Read the model definition and answer for the solid it produces. Units are mm, in the model's axes. Coordinates: 2 decimals unless noted, no trailing zeros. Write each loop counter-clockwise with the first axis right and the second up, starting at its lowest first coordinate (ties: lowest second). Pieces come first, ordered by that corner, then holes.
1) The part is cut by section B-B (x = 0). Determine the outline of the cut face in (y, z), then the cut area to 3 significant figures.
2) The part is cut by section A-A (y = -1.7). Determine the outline of the cut face in (x, z).
3) The part is cut by section D-D (x = 16). Determine the outline of the cut face in (y, z), then the cut area to 3 significant figures.
4) Each of these flat-tipped pins is pushed along its axis until it touches: pin 1 Ø1.1 at (y, z) = (-1.5, 15) entering from -X; pin 2 Ø6 at (x, z) = (-13.5, -16) entering from -Y; pin 3 Ø0.5 at (x, y) = (-0.5, -1) entering from +Z. Where does it stop, or does it pass through?
5) The part is cut by section C-C (z = 0). Determine the outline of the cut face in (x, y).
6) Find the intervals of material crossed by line 1 (Z direction, x = 1, y = -1.75); line 2 (Y direction, x = -15, z = 2); line 3 (X direction, y = 0.35, z = 18.5), in increasing order.
from build123d import *

# Parameters (mm, degrees)
FRONT_W       = 20.95
FRONT_H       = 1
SKETCH1_W     = 4
SKETCH1_H     = 1
HOLDERS_DEPTH = 1.8


with BuildPart() as part:
    # Front → Base (revolve)
    with BuildSketch(Plane.XY, mode=Mode.PRIVATE) as base_sk:
        with Locations((-10.475, 0)):
            Rectangle(FRONT_W, FRONT_H)
    revolve(base_sk.sketch.rotate(Axis((0, 0, 0), (0, 1, 0)), 270), axis=Axis((0, 0, 0), (0, 1, 0)))

    # Sketch1 → Holders (add)
    with BuildSketch(Plane.XZ.offset(0.5)):
        with Locations((0, 15)):
            Rectangle(SKETCH1_W, SKETCH1_H)
        with Locations((0, -15)):
            Rectangle(SKETCH1_W, SKETCH1_H)
    extrude(amount=HOLDERS_DEPTH)


solid = part.part
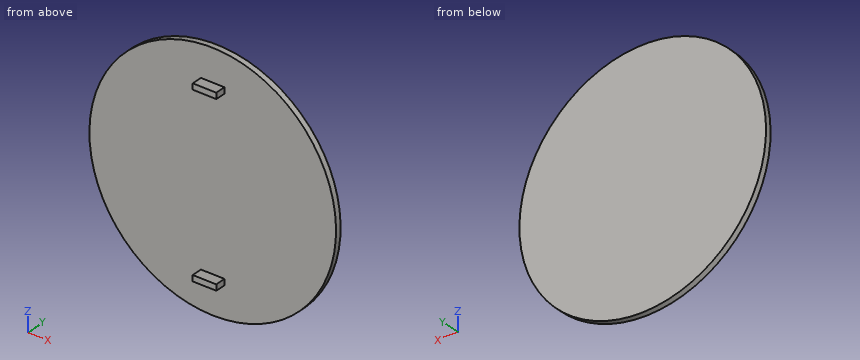
Reported:
1. outline: (-2.3, -15.5) - (-0.5, -15.5) - (-0.5, -20.95) - (0.5, -20.95) - (0.5, 20.95) - (-0.5, 20.95) - (-0.5, 15.5) - (-2.3, 15.5) - (-2.3, 14.5) - (-0.5, 14.5) - (-0.5, -14.5) - (-2.3, -14.5) - close
1. area: 45.5 mm2
2. outline: (-2, -15.5) - (2, -15.5) - (2, -14.5) - (-2, -14.5) - close; (-2, 14.5) - (2, 14.5) - (2, 15.5) - (-2, 15.5) - close
3. outline: (-0.5, -13.52) - (0.5, -13.52) - (0.5, 13.52) - (-0.5, 13.52) - close
3. area: 27.0 mm2
4. pin 1: stops at x = -2
4. pin 2: stops at y = -0.5
4. pin 3: stops at z = 15.5
5. outline: (-20.95, -0.5) - (20.95, -0.5) - (20.95, 0.5) - (-20.95, 0.5) - close
6. line 1: z = -15.5 to -14.5, 14.5 to 15.5
6. line 2: y = -0.5 to 0.5
6. line 3: x = -9.83 to 9.83
